Could you check a few things on this model? Use its own coordinates, in mm. Face numbers are marked on the shaded views. A direction names the side the tool comes from. Coordinates: 2 decimals unless noted, no trailing zeros. Write each loop counter-clockwise with the first axis right and the second up, starting at its lowest first coordinate (ties: lowest second). Pieces come first, ordered by that corner, then holes. Notation, with made-up numbers: M 18.5,-30 L 43.5,-30 A24 cw 43.5,-2 Z; hole C 79,45 d7. An arc over 180 degrees is marked long. Write item = value, one per line.
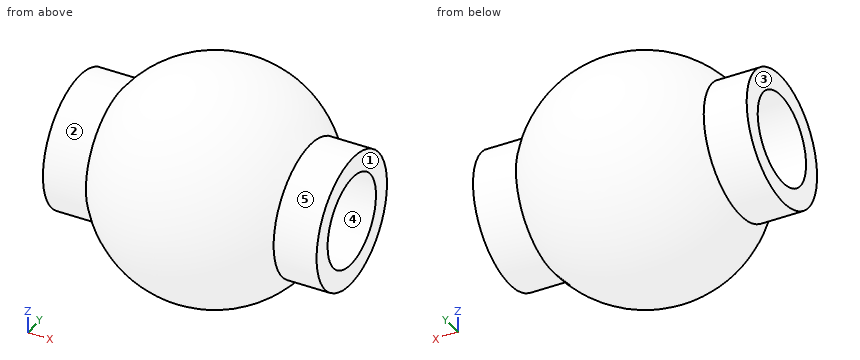
Autodesk Inventor part; units mm, degrees
ref_plane "YZ Plane" through (0, 0, 0) normal (1, 0, 0) x (0, 1, 0)
ref_plane "XZ Plane" through (0, 0, 0) normal (0, 1, 0) x (-1, 0, 0)
ref_plane "XY Plane" through (0, 0, 0) normal (0, 0, 1) x (1, 0, 0)
sketch "Sketch1" plane through (0, 0, 0) normal (0, 0, 1) x (1, 0, 0)
  arc A0 (0, -2.9) -> (0, 2.9) centre (0, 0) ccw
  line L0 (0, 0) -> (0, 2.9)
  line L1 (0, 0) -> (0, -2.9)
  dimension "d0" = 5.8
revolve "Revolution1" add sketch "Sketch1" angle 360 about axis through (0, 0, 0) along (0, 1, 0)
sketch "Sketch3" plane through (0, 0, 0) normal (1, 0, 0) x (0, 1, 0)
  circle A0 centre (0, 0) radius 1.675
  dimension "d4" = 3.35
extrude "Extrusion1" add sketch "Sketch3" along normal mid plane 6.9
sketch "Sketch4" plane through (3.45, 0, 0) normal (1, 0, 0) x (0, 0, -1)
  circle A0 centre (0, 0) radius 1.15
  dimension "d7" = 2.3
extrude "Extrusion2" cut sketch "Sketch4" against normal blind 6.9
properties part number "RCT-H017_lower_linkage_ball_stud"
Item 1: Imagine slicing it at A-A (y = 0). Write out the boundary of the cut face in (x, z) (3 decimals).
Numbers:
outline = M -3.45,-1.675 L -2.367,-1.675 A2.9 ccw 2.367,-1.675 L 3.45,-1.675 L 3.45,-1.15 L -3.45,-1.15 Z; M -3.45,1.15 L 3.45,1.15 L 3.45,1.675 L 2.367,1.675 A2.9 ccw -2.367,1.675 L -3.45,1.675 Z
Item 2: If we mould it in two halves opening along Z, with no side actions, what happens to the marked faces 3, 4 and 5? For each: pulls with the +Z half, pulls with the -Z half, needs draft (parallel to the pull), parting line crosses it, or undercut.
Numbers:
face_3 = needs draft
face_4 = undercut
face_5 = parting line crosses it
Item 3: Imagine slicing it at D-D (y = 1.3). Write out the boundary of the cut face in (x, z).
Numbers:
outline = M -3.45,-1.06 L -2.37,-1.06 A2.59 ccw 2.37,-1.06 L 3.45,-1.06 L 3.45,1.06 L 2.37,1.06 A2.59 ccw -2.37,1.06 L -3.45,1.06 Z
Item 4: I'm going to push flat-ended pins straight in: P1, Ø1, axis at x = 2, y = 1, coming from the -Z side; P2, Ø3, axis at x = -1.5, y = -2.5, coming from the +Z side. Where does each tip first touch, or does it pass through?
Numbers:
P1 = -2.32
P2 = 2.53
Item 5: Imagine slicing it at C-C (x = 2). Write out the boundary of the cut face in (y, z).
Numbers:
outline = C 0,0 d4.2; hole C 0,0 d2.3
Item 6: If I drill on line 1 along Y through (x, z) = (-2, 0); line 2 along Y through (x, z) = (-3, -1); line 3 along X through (y, z) = (1.2, 2.4), over which ranges is the centre line in solid material (lowest first)?
Numbers:
line_1 = -2.1 to -1.15, 1.15 to 2.1
line_2 = -1.34 to -0.57, 0.57 to 1.34
line_3 = -1.1 to 1.1
Item 7: For the marked faces 1 and 2, which set-ups out of +Z, -Z, +X, -X, +Y, -Y let a thin tool reach every point of the face, with its end or its side?
Numbers:
face_1 = +Z, -Z, +X, +Y, -Y
face_2 = -X
